from build123d import *

# Parameters (mm, degrees)
ESQUISSE1_R        = 5
ESQUISSE1_R_2      = 2
BOSS_EXTRU_1_DEPTH = 4


with BuildPart() as part:
    # Esquisse1 → Boss.-Extru.1 (new body)
    with BuildSketch(Plane.XY):
        with BuildLine():
            Line((33, -5), (33, 5))
            Line((33, 5), (29, 5))
            Line((29, 5), (29, 15))
            ThreePointArc((29, 15), (21.811905433, 16.204525755), (15.409139214, 19.686503719))
            ThreePointArc((15.409139214, 19.686503719), (0, 25), (-15.409139214, 19.686503719))
            ThreePointArc((-15.409139214, 19.686503719), (-21.811905433, 16.204525755), (-29, 15))
            Line((-29, 15), (-29, 5))
            Line((-29, 5), (-33, 5))
            Line((-33, 5), (-33, -5))
            Line((-33, -5), (-29, -5))
            Line((-29, -5), (-29, -15))
            ThreePointArc((-29, -15), (-21.811905433, -16.204525755), (-15.409139214, -19.686503719))
            ThreePointArc((-15.409139214, -19.686503719), (0, -25), (15.409139214, -19.686503719))
            ThreePointArc((15.409139214, -19.686503719), (21.811905433, -16.204525755), (29, -15))
            Line((29, -15), (29, -5))
            Line((29, -5), (33, -5))
        make_face()
        Circle(ESQUISSE1_R, mode=Mode.SUBTRACT)
        with Locations((-8.838834765, 8.838834765)):
            Circle(ESQUISSE1_R_2, mode=Mode.SUBTRACT)
        with Locations((8.838834765, 8.838834765)):
            Circle(ESQUISSE1_R_2, mode=Mode.SUBTRACT)
        with Locations((8.838834765, -8.838834765)):
            Circle(ESQUISSE1_R_2, mode=Mode.SUBTRACT)
        with Locations((-8.838834765, -8.838834765)):
            Circle(ESQUISSE1_R_2, mode=Mode.SUBTRACT)
    extrude(amount=BOSS_EXTRU_1_DEPTH)


solid = part.part
Design review of the part built by this model. Coordinates are the model's own, in mm. A direction names the side the tool comes from. Give positions to 0.01 mm unless a question says otherwise; leave off trailing zeros. Loops run counter-clockwise (first coordinate to the right, second up) from the corner with the lowest first, then second, coordinate; pieces in that order, holes last. Notation, with made-up numbers: M 27.5,89 L 46.5,89 A30 ccw 46.5,127 Z; hole C 27,27 d5. An arc over 180 degrees is marked long. Write item = value, one per line.
Q1. Draft analysis for pull direction X (two halves, no side actions). For faces 4 (the cylindrical face through (7.365, 10.191, 1.972)), 5 (the cylindrical face through (0, -25, 2)), 6 (the flat face through (31, 5, 2)), 7 (the cylindrical face through (-10.313, 10.191, 1.972)), state which applies: +X half, -X half, draft (parallel to the pull), parting line (faces both ways), or undercut.
Output values:
face_4 = undercut
face_5 = parting line
face_6 = draft
face_7 = undercut
Q2. We need section D-D (y = -10). Give the boundary of the cut face in (x, z), plus the area to 3 significant figures.
Output values:
outline = M -29,0 L -10.47,0 L -10.47,4 L -29,4 Z; M -7.21,0 L 7.21,0 L 7.21,4 L -7.21,4 Z; M 10.47,0 L 29,0 L 29,4 L 10.47,4 Z
area = 206 mm^2
Q3. We need section A-A (y = 0). Give the boundary of the cut face in (x, z).
Output values:
outline = M -33,0 L -5,0 L -5,4 L -33,4 Z; M 5,0 L 33,0 L 33,4 L 5,4 Z
Q4. For faces 1 (the flat face through (31, -5, 2)), 2 (the flat face through (-29, -10, 2)), 3 (the flat face through (-29, 10, 2)), list the 3-axis set-ups (+Z, -Z, +X, -X, +Y, -Y) from which the entire face can be reached by the end or side of a thin tool; tool diameter is ignored.
Output values:
face_1 = +Z, -Z, +X, -Y
face_2 = +Z, -Z, -X, -Y
face_3 = +Z, -Z, -X, +Y
Q5. Insertion check: pin 1 (2 mm diameter, centred on x = 16.5, z = 0.5, fed in from -Y); pin 2 (2 mm diameter, centred on y = -12.5, z = 2, fed in from +X); pin 3 (1.2 mm diameter, centred on x = 31.5, z = 3, fed in from -Y); pin 4 (5 mm diameter, centred on x = 8.84, y = 8.84, fed in from -Z). Each pin has a flat end and moves straight along its axis. Give the tip position at first contact, or say it passes through.
Output values:
pin_1 = -19.62
pin_2 = 29
pin_3 = -5
pin_4 = 0
Q6. We need section C-C (z = 2.55). Give the boundary of the cut face in (x, y), plus the area to 3 significant figures.
Output values:
outline = M -33,-5 L -29,-5 L -29,-15 A22.05 cw -15.41,-19.69 A25 ccw 15.41,-19.69 A22.05 cw 29,-15 L 29,-5 L 33,-5 L 33,5 L 29,5 L 29,15 A22.05 cw 15.41,19.69 A25 ccw -15.41,19.69 A22.05 cw -29,15 L -29,5 L -33,5 Z; hole C -8.84,-8.84 d4; hole C -8.84,8.84 d4; hole C 0,0 d10; hole C 8.84,-8.84 d4; hole C 8.84,8.84 d4
area = 2,280 mm^2
Q7. To check wall thickness, follow line 1 (X direction, y = 9, z = 2.05); line 2 (X direction, y = 10, z = 1.1); line 3 (Y direction, x = -3.5, z = 3.55). State the ranges of each line that lie inside material, in increasing order. Write a range as [from, to].
Output values:
line_1 = [-29, -10.83], [-6.85, 6.85], [10.83, 29]
line_2 = [-29, -10.47], [-7.21, 7.21], [10.47, 29]
line_3 = [-24.75, -3.57], [3.57, 24.75]
Q8. We need section B-B (x = 0). Give the boundary of the cut face in (y, z), plus the area to 3 significant figures.
Output values:
outline = M -25,0 L -5,0 L -5,4 L -25,4 Z; M 5,0 L 25,0 L 25,4 L 5,4 Z
area = 160 mm^2
